Source: CAD feature listing. Evaluate the final solid. Frame: model axes, mm. Face numbers are marked on the shaded views. A direction names the side the tool comes from. Coordinates: 2 decimals unless noted, no trailing zeros. Order: outer loops, then holes, each group sorted by start corner. A loop starts at its lowest first (then second) coordinate and runs counter-clockwise, first axis right, second up. Notation, with made-up numbers: (80, 12.5) - (106, 12.5) arc R23 cw to (106, 46.5) - close; hole circle Ø4 at (-1.75, 59). An arc over 180 degrees is marked (long way). One line per question, with ' | ' between items.
from build123d import *

# Parameters (mm, degrees)
EXTRUDE_1_DEPTH     = 10
SKETCH_4_R          = 2
CUT_EXTRUDE_1_DEPTH = 10
SKETCH_2_R          = 2
CUT_EXTRUDE_2_DEPTH = 20
FILLET_2_R          = 0.5
FILLET_3_R          = 3
FILLET_4_R          = 1


with BuildPart() as part:
    # 草图1 → 凸台-拉伸1 (new body)
    with BuildSketch(Plane.XY):
        with BuildLine():
            Line((-13, 0), (-13, -11))
            ThreePointArc((-13, -11), (-13.585786438, -12.414213562), (-15, -13))
            Line((-15, -13), (-15.5, -13))
            ThreePointArc((-15.5, -13), (-15.853553391, -12.853553391), (-16, -12.5))
            Line((-16, -12.5), (-16, 3))
            Line((-16, 3), (-0.5, 3))
            ThreePointArc((-0.5, 3), (-0.146446609, 2.853553391), (0, 2.5))
            Line((0, 2.5), (0, 2))
            ThreePointArc((0, 2), (-0.585786438, 0.585786438), (-2, 0))
            Line((-2, 0), (-13, 0))
        make_face()
    extrude(amount=EXTRUDE_1_DEPTH)

    # 草图4 → 切除-拉伸1 (cut)
    with BuildSketch(Plane(origin=(0, 0, 0), x_dir=(1, 0, 0), z_dir=(0, 1, 0))):
        with Locations((-5, -5)):
            Circle(SKETCH_4_R)
    extrude(amount=CUT_EXTRUDE_1_DEPTH, mode=Mode.SUBTRACT)

    # 草图2 → 切除-拉伸2 (cut)
    with BuildSketch(Plane(origin=(-13, 0, 0), x_dir=(0, 0, -1), z_dir=(1, 0, 0))):
        with Locations((-5, -8)):
            Circle(SKETCH_2_R)
    extrude(amount=-CUT_EXTRUDE_2_DEPTH, mode=Mode.SUBTRACT)

    # 圆角2
    fillet_2_edges = [part.edges().sort_by_distance(p)[0] for p in [
        (-7, 0, 5),
        (-13, -8, 7),
    ]]
    fillet(fillet_2_edges, radius=FILLET_2_R)

    # 圆角3
    fillet_3_edges = [part.edges().sort_by_distance(p)[0] for p in [
        (-13, 0, 5),
    ]]
    fillet(fillet_3_edges, radius=FILLET_3_R)

    # 圆角4
    fillet_4_edges = [part.edges().sort_by_distance(p)[0] for p in [
        (-16, 3, 5),
    ]]
    fillet(fillet_4_edges, radius=FILLET_4_R)


solid = part.part
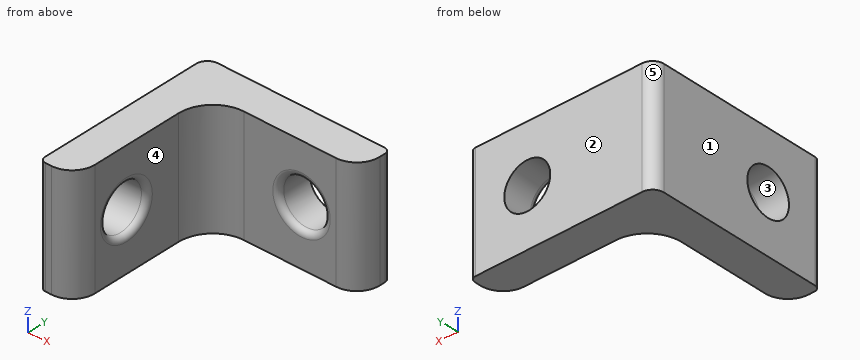
(1) Cut plane C-C (y = -8). Return the cut outline in (x, z), and give its area (3 significant figures).
Taken from the geometry:
outline: (-16, 0) - (-13, 0) - (-13, 2.5) arc R0.5 ccw to (-13.5, 3) - (-16, 3) - close; (-16, 7) - (-13.5, 7) arc R0.5 ccw to (-13, 7.5) - (-13, 10) - (-16, 10) - close | area: 17.9 mm²
(2) Cut plane A-A (x = -5). Return the cut outline in (y, z).
Taken from the geometry:
outline: (0, 0) - (3, 0) - (3, 3) - (0.5, 3) arc R0.5 ccw to (0, 2.5) - close; (0, 7.5) arc R0.5 ccw to (0.5, 7) - (3, 7) - (3, 10) - (0, 10) - close
(3) Pin query (flat end, axial travel): P1, Ø3, axis at x = -5, z = 5, coming from the +Y side (1 decimal); P2, Ø2.5, axis at x = -6, z = 5, coming from the -Y side; P3, Ø1, axis at y = -4, z = 7, coming from the +X side. Return the tip coordinate at first contact, or that it passes through.
Taken from the geometry:
P1: passes through | P2: stops at y = 0.07 | P3: stops at x = -13
(4) Cut plane D-D (z = 9.75). Return the cut outline in (x, y).
Taken from the geometry:
outline: (-16, -12.5) arc R0.5 ccw to (-15.5, -13) - (-15, -13) arc R2 ccw to (-13, -11) - (-13, -3) arc R3 cw to (-10, 0) - (-2, 0) arc R2 ccw to (0, 2) - (0, 2.5) arc R0.5 ccw to (-0.5, 3) - (-15, 3) arc R1 ccw to (-16, 2) - close
(5) Pull-direction query (Y, two-part tool) for the marked faces 1, 2 and 3; classes: pulls with the +Y half, pulls with the -Y half, needs draft (parallel to the pull), parting line crosses it, or undercut.
Taken from the geometry:
face 1: needs draft | face 2: pulls with the +Y half | face 3: undercut
(6) Cut plane B-B (z = 5). Return the cut outline in (x, y), and give its area (3 significant figures).
Taken from the geometry:
outline: (-16, -12.5) arc R0.5 ccw to (-15.5, -13) - (-15, -13) arc R2 ccw to (-13, -11) - (-13, -10.5) arc R0.5 ccw to (-13.5, -10) - (-16, -10) - close; (-16, -6) - (-13.5, -6) arc R0.5 ccw to (-13, -5.5) - (-13, -3) arc R3 cw to (-10, 0) - (-7.5, 0) arc R0.5 ccw to (-7, 0.5) - (-7, 3) - (-15, 3) arc R1 ccw to (-16, 2) - close; (-3, 0.5) arc R0.5 ccw to (-2.5, 0) - (-2, 0) arc R2 ccw to (0, 2) - (0, 2.5) arc R0.5 ccw to (-0.5, 3) - (-3, 3) - close | area: 62.7 mm²
(7) Set-up query: the marked faces 4 and 5. Return all of +Z, -Z, +X, -X, +Y, -Y with unobstructed straight access to the full face (end or side cutting, diameter ignored); none if empty.
Taken from the geometry:
face 4: +Z, -Z, +X, -Y | face 5: +Z, -Z, -X, +Y
(8) Material intervals for L1, parallel to Z at x = -5, y = 2.3; L2, parallel to Y at x = -8, z = 6; L3, parallel to X at y = 1.25, z = 5.25, sorted ascending. Write a range as from..to.
Taken from the geometry:
L1: z = 0..3, 7..10 | L2: y = 0..3 | L3: x = -16..-6.98, -3.02..-0.15
